The model under review builds one solid part; all positions refer to its coordinate system, in mm. Face numbers are marked on the shaded views. A direction names the side the tool comes from. Coordinates: 2 decimals unless noted, no trailing zeros. Order: outer loops, then holes, each group sorted by start corner. A loop starts at its lowest first (then second) coordinate and runs counter-clockwise, first axis right, second up.
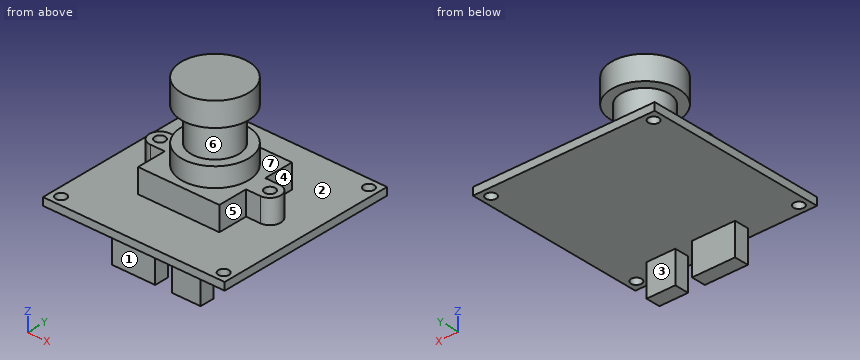
```python
from build123d import *

# Parameters (mm, degrees)
SKETCH_1_W      = 38
SKETCH_1_H      = 38
SKETCH_1_R      = 1.1
EXTRUDE_2_DEPTH = 1.6
SKETCH_1_4_W    = 17
SKETCH_1_4_H    = 17
SKETCH_1_4_R    = 1.1
EXTRUDE_3_DEPTH = 5
EXTRUDE_START   = -1.6
SKETCH_4_W      = 6
SKETCH_4_H      = 3
SKETCH_4_W_2    = 9
EXTRUDE_4_DEPTH = 8.3


with BuildPart() as part:
    # 草图1 → 凸台-拉伸2 (new body)
    with BuildSketch(Plane.XY):
        Rectangle(SKETCH_1_W, SKETCH_1_H)
        with Locations((-17, 17)):
            Circle(SKETCH_1_R, mode=Mode.SUBTRACT)
        with Locations((17, 17)):
            Circle(SKETCH_1_R, mode=Mode.SUBTRACT)
        with Locations((17, -17)):
            Circle(SKETCH_1_R, mode=Mode.SUBTRACT)
        with Locations((-17, -17)):
            Circle(SKETCH_1_R, mode=Mode.SUBTRACT)
    extrude(amount=-EXTRUDE_2_DEPTH)

    # 草图1<4> → 凸台-拉伸3 (add)
    # profile 1 of 2: a face of its own
    with BuildSketch(Plane.XY):
        Rectangle(SKETCH_1_4_W, SKETCH_1_4_H)
    # profile 2 of 2: a face of its own
    with BuildSketch(Plane.XY):
        with BuildLine():
            Line((-11.5, 2.25), (11.5, 2.25))
            ThreePointArc((11.5, 2.25), (13.75, 0), (11.5, -2.25))
            Line((11.5, -2.25), (-11.5, -2.25))
            ThreePointArc((-11.5, -2.25), (-13.75, 0), (-11.5, 2.25))
        make_face()
        with Locations((11.5, 0)):
            Circle(SKETCH_1_4_R, mode=Mode.SUBTRACT)
        with Locations((-11.5, 0)):
            Circle(SKETCH_1_4_R, mode=Mode.SUBTRACT)
    extrude(amount=EXTRUDE_3_DEPTH)

    # 草图3 → 旋转3 (revolve)
    with BuildSketch(Plane(origin=(0, 0, 0), x_dir=(0, 0, -1), z_dir=(1, 0, 0))):
        Polygon((-5, 0), (-9, 0), (-16, 0), (-21, 0), (-21, 7), (-16, 7), (-16, 5), (-9, 5), (-9, 7), (-5, 7), align=None)
    revolve(axis=Axis((0, 0, 5), (0, 0, 1)))

    # 草图4 → 凸台-拉伸4 (add)
    with BuildSketch(Plane(origin=(0, 0, -1.6), x_dir=(-1, 0, 0), z_dir=(0, 0, -1)).offset(EXTRUDE_START)):
        with Locations((-9, -15.3)):
            Rectangle(SKETCH_4_W, SKETCH_4_H)
        with Locations((2, -15.3)):
            Rectangle(SKETCH_4_W_2, SKETCH_4_H)
    extrude(amount=EXTRUDE_4_DEPTH)


solid = part.part
```
(1) We need section B-B, the plane y = 0. Write out the cut boundary in (x, z).
A:
outline: (-19, -1.6) - (19, -1.6) - (19, 0) - (13.75, 0) - (13.75, 5) - (12.6, 5) - (12.6, 0) - (10.4, 0) - (10.4, 5) - (7, 5) - (7, 9) - (5, 9) - (5, 16) - (7, 16) - (7, 21) - (-7, 21) - (-7, 16) - (-5, 16) - (-5, 9) - (-7, 9) - (-7, 5) - (-10.4, 5) - (-10.4, 0) - (-12.6, 0) - (-12.6, 5) - (-13.75, 5) - (-13.75, 0) - (-19, 0) - close
(2) We need section D-D, the plane x = 0. Write out the cut boundary in (y, z).
A:
outline: (-19, -1.6) - (-16.8, -1.6) - (-16.8, -8.3) - (-13.8, -8.3) - (-13.8, -1.6) - (19, -1.6) - (19, 0) - (8.5, 0) - (8.5, 5) - (7, 5) - (7, 9) - (5, 9) - (5, 16) - (7, 16) - (7, 21) - (-7, 21) - (-7, 16) - (-5, 16) - (-5, 9) - (-7, 9) - (-7, 5) - (-8.5, 5) - (-8.5, 0) - (-19, 0) - close
(3) Machinability: for the marked faces 1, 2, 3 and 4, which of the approach directions +Z, -Z, +X, -X, +Y, -Y give a long, thin tool a straight path to every point of the face, cutting with its end or side? Answer none if there is none.
A:
face 1: -Z, +X, -X, -Y
face 2: +Z
face 3: -Z, +X, -X, +Y
face 4: +Z, +X, +Y
(4) For pin 1 Ø1.3 at (x, y) = (17, -17) entering from -Z; pin 2 Ø2.5 at (x, y) = (-11.5, 0.5) entering from +Z; pin 3 Ø8 at (x, y) = (4, -15) entering from +Z; pin 4 Ø5.5 at (x, z) = (0, -5) entering from -Y, all flat-tipped, find the tip position at first contact; note any pin that passes through.
A:
pin 1: passes through
pin 2: stops at z = 5
pin 3: stops at z = 0
pin 4: stops at y = -16.8
(5) Wall thickness on probe 1 along Y at (x, z) = (-17, -1); probe 2 along X at (y, z) = (1, 2.75); probe 3 along Z at (x, y) = (3.5, -4): over which ranges is each line inside the solid? List them lowest first.
A:
probe 1: y = -19 to -18.1, -15.9 to 15.9, 18.1 to 19
probe 2: x = -13.52 to -11.96, -11.04 to 11.04, 11.96 to 13.52
probe 3: z = -1.6 to 9, 16 to 21
(6) We need section A-A, the plane z = -3.75. Write out the cut boundary in (x, y), and give its area (3 significant figures).
A:
outline: (-6.5, -16.8) - (2.5, -16.8) - (2.5, -13.8) - (-6.5, -13.8) - close; (6, -16.8) - (12, -16.8) - (12, -13.8) - (6, -13.8) - close
area: 45.0 mm2
(7) Draft analysis for pull direction Z (two halves, no side actions). For the marked faces 5, 6 and 7, state which applies: released by +Z, released by -Z, zero draft, split by the parting line, or undercut.
A:
face 5: zero draft
face 6: undercut
face 7: released by +Z
(8) We need section C-C, the plane x = -17. Write out the cut boundary in (y, z), and give its area (3 significant figures).
A:
outline: (-19, -1.6) - (-18.1, -1.6) - (-18.1, 0) - (-19, 0) - close; (-15.9, -1.6) - (15.9, -1.6) - (15.9, 0) - (-15.9, 0) - close; (18.1, -1.6) - (19, -1.6) - (19, 0) - (18.1, 0) - close
area: 53.8 mm2
